Autodesk Inventor part; units mm, degrees
ref_plane "YZ Plane" through (0, 0, 0) normal (1, 0, 0) x (0, 1, 0)
ref_plane "XZ Plane" through (0, 0, 0) normal (0, 1, 0) x (-1, 0, 0)
ref_plane "XY Plane" through (0, 0, 0) normal (0, 0, 1) x (1, 0, 0)
sketch "Sketch1" plane through (0, 0, 0) normal (0, 0, 1) x (1, 0, 0)
  line L0 (-15, 55) -> (15, 55)
  line L1 (15, 55) -> (15, -55)
  line L2 (15, -55) -> (-15, -55)
  line L3 (-15, -55) -> (-15, 55)
  line L4 (-15, 55) -> (15, -55) construction
  line L5 (15, 55) -> (-15, -55) construction
  line L6 (-15, 19) -> (-75, 19)
  line L7 (-75, 19) -> (-75, -19)
  line L8 (-75, -19) -> (-15, -19)
  line L9 (-15, -19) -> (-15, 19)
  arc A0 (-51, 19) -> (-15, 55) centre (-51, 55) ccw
  arc A1 (-15, -55) -> (-51, -19) centre (-51, -55) ccw
  circle A2 centre (0, 40) radius 5.5
  circle A3 centre (0, -40) radius 5.5
  line L10 (0, 0) -> (15, 0) construction
  point P0 (-75, 0)
  dimension "d157" = 30
  dimension "d158" = 110
  dimension "d159" = 38
  dimension "d160" = 80
  dimension "d161" = 11
  dimension "d162" = 60
extrude "Plate3" add sketch "Sketch1" along normal blind 3
fillet "Corner Round2" radius 6 4 edges at (-15, 55, 1.5) (15, 55, 1.5) (-15, -55, 1.5) (15, -55, 1.5)
equation "\"BendReliefWidth\" = Thickness"
equation "\"BendReliefDepth\" = 0.5 * Thickness"
equation "\"CornerReliefSize\" = 4 * Thickness"
equation "\"MinimumRemnant\" = 2 * Thickness"
equation "\"GapSize\" = Thickness"
properties part number "MSC 815 wall inner" material "AISI304"
The model under review builds one solid part; all positions refer to its coordinate system, in mm. A direction names the side the tool comes from. Give positions to 0.01 mm unless a question says otherwise; leave off trailing zeros. Order: outer loops, then holes, each group sorted by start corner. A loop starts at its lowest first (then second) coordinate and runs counter-clockwise, first axis right, second up. Notation, with made-up numbers: (-8.75, 26.25) -> (6.25, 26.25) arc R17 cw to (6.25, 49.25) -> close; hole circle Ø5 at (9, 78.5). An arc over 180 degrees is marked (long way). Write item = value, one per line. Start each with the question number.
(1) For pin 1 Ø6.5 at (x, y) = (0, -40) entering from +Z; pin 2 Ø0.9 at (x, z) = (-58, 1.5) entering from +Y, all flat-tipped, find the tip position at first contact; note any pin that passes through.
(2) Take a section at A-A (x = 0). Write out the cut boundary in (y, z), plus the area to 3 significant figures.
(3) Take a section at D-D (y = -40). Write out the cut boundary in (x, z), plus the area to 3 significant figures.
(4) For L1, parallel to Y at x = 0, z = 2.25; L2, parallel to Y at x = -2, z = 1.75; L3, parallel to X at y = -39, z = 0.75, list the stretches that pass through material, from the lowest coordinate up. Write a range as from..to.
(5) Take a section at B-B (z = 1.35). Write out the cut boundary in (x, y).
(6) Take a section at C-C (y = 41.5). Write out the cut boundary in (x, z), plus the area to 3 significant figures.
(7) Draft analysis for pull direction Y (two halves, no side actions). For faces 1 (the cylindrical face through (13.289, 53.196, 1.521)), 2 (the cylindrical face through (-13.4, -53.5, 1.5)), 3 (the flat face through (15, 1, 1)), 4 (the cylindrical face through (-0.716, 34.547, 1.479)), state which applies: +Y half, -Y half, draft (parallel to the pull), parting line (faces both ways), or undercut.
(8) Tool access review of faces 5 (the flat face through (-63, 19, 1)), 6 (the cylindrical face through (13.196, -53.289, 1.521)), 7 (the flat face through (-63, -19, 1)): name each direction out of +Z, -Z, +X, -X, +Y, -Y from which nothing blocks a thin tool from reaching the whole face with its end or side.
Returned:
q1.pin_1 = through
q1.pin_2 = 19
q2.outline = (-55, 0) -> (-45.5, 0) -> (-45.5, 3) -> (-55, 3) -> close; (-34.5, 0) -> (34.5, 0) -> (34.5, 3) -> (-34.5, 3) -> close; (45.5, 0) -> (55, 0) -> (55, 3) -> (45.5, 3) -> close
q2.area = 264 mm²
q3.outline = (-18.27, 0) -> (-5.5, 0) -> (-5.5, 3) -> (-18.27, 3) -> close; (5.5, 0) -> (15, 0) -> (15, 3) -> (5.5, 3) -> close
q3.area = 66.8 mm²
q4.L1 = -55..-45.5, -34.5..34.5, 45.5..55
q4.L2 = -55..-45.12, -34.88..34.88, 45.12..55
q4.L3 = -18.75..-5.41, 5.41..15
q5.outline = (-75, -19) -> (-51, -19) arc R36 cw to (-15.37, -49.86) arc R6 ccw to (-9.43, -55) -> (9, -55) arc R6 ccw to (15, -49) -> (15, 49) arc R6 ccw to (9, 55) -> (-9.43, 55) arc R6 ccw to (-15.37, 49.86) arc R36 cw to (-51, 19) -> (-75, 19) -> close; hole circle Ø11 at (0, -40); hole circle Ø11 at (0, 40)
q6.outline = (-17.63, 0) -> (-5.29, 0) -> (-5.29, 3) -> (-17.63, 3) -> close; (5.29, 0) -> (15, 0) -> (15, 3) -> (5.29, 3) -> close
q6.area = 66.1 mm²
q7.face_1 = +Y half
q7.face_2 = -Y half
q7.face_3 = draft
q7.face_4 = undercut
q8.face_5 = +Z, -Z, -X, +Y
q8.face_6 = +Z, -Z, +X, -Y
q8.face_7 = +Z, -Z, -X, -Y
